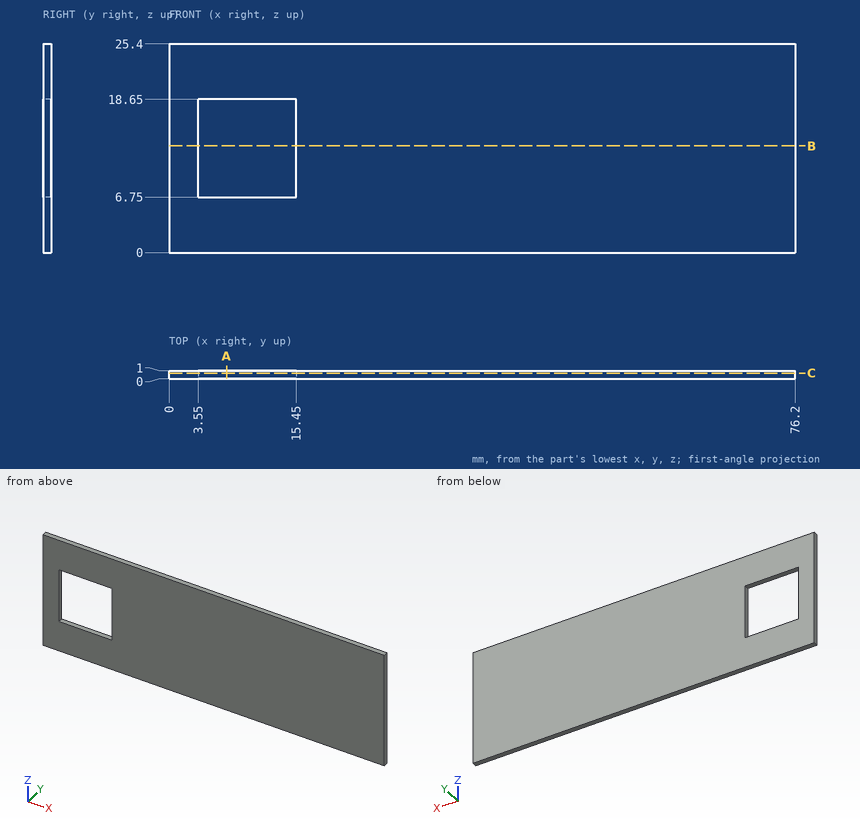
The figure shows three views and two pictorial views of one solid part (mm, origin at its lowest corner). Answer the questions. Coordinates: 2 decimals unless noted, no trailing zeros. Loops run counter-clockwise (first coordinate to the right, second up) from the corner with the lowest first, then second, coordinate; pieces in that order, holes last. Notation, with made-up numbers: (-32, 43.25) -> (-22, 43.25) arc R19 cw to (-22, 66.25) -> close; hole circle Ø1 at (64, 70). An arc over 180 degrees is marked (long way). Use one line per item in the form item = value. Start each with the question number.
Item 1: The part is cut by section B-B on z = 13. Determine the outline of the cut face in (x, y), then the cut area to 3 significant figures.
Item 2: The part is cut by section C-C on y = 0.7. Determine the outline of the cut face in (x, z).
Item 3: The part is cut by section A-A on x = 7. Determine the outline of the cut face in (y, z).
Item 4: Consider L1, parallel to X at y = 0.1, z = 14; L2, parallel to Z at x = 12, y = 0.4. Determine where each line is inside the solid, lowest interval first. Write a range as [from, to].
Answer key:
q1.outline = (0, 0) -> (3.55, 0) -> (3.55, 1) -> (0, 1) -> close; (15.45, 0) -> (76.2, 0) -> (76.2, 1) -> (15.45, 1) -> close
q1.area = 64.3 mm2
q2.outline = (0, 0) -> (76.2, 0) -> (76.2, 25.4) -> (0, 25.4) -> close; hole (3.55, 6.75) -> (15.45, 6.75) -> (15.45, 18.65) -> (3.55, 18.65) -> close
q3.outline = (0, 0) -> (1, 0) -> (1, 6.75) -> (0, 6.75) -> close; (0, 18.65) -> (1, 18.65) -> (1, 25.4) -> (0, 25.4) -> close
q4.L1 = [0, 3.55], [15.45, 76.2]
q4.L2 = [0, 6.75], [18.65, 25.4]
